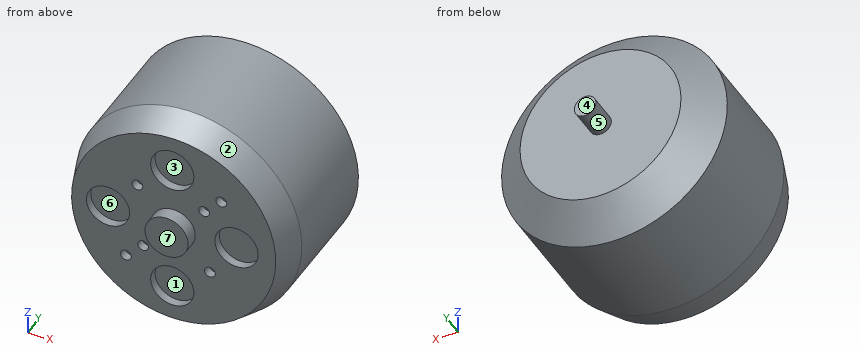
from build123d import *

# Parameters (mm, degrees)
SKETCH1_R           = 20.9
BOSS_EXTRUDE1_DEPTH = 30.75
CHAMFER1_SIZE       = 5
CHAMFER1_SIZE2      = 6
CHAMFER2_SIZE       = 2
CHAMFER2_SIZE2      = 5.494954839
SKETCH2_R           = 2
BOSS_EXTRUDE2_DEPTH = 5.5
SKETCH3_R           = 4
BOSS_EXTRUDE3_DEPTH = 2.55
SKETCH4_R           = 4
SKETCH4_R_2         = 1
CUT_EXTRUDE1_DEPTH  = 1.5875


with BuildPart() as part:
    # Sketch1 → Boss-Extrude1 (new body)
    with BuildSketch(Plane(origin=(0, 0, 0), x_dir=(1, 0, 0), z_dir=(0, 1, 0))):
        with Locations(Location((-5.649057894, -5.328088696, 0), (0, 0, 270))):
            Circle(SKETCH1_R)
    extrude(amount=BOSS_EXTRUDE1_DEPTH)

    # Chamfer1
    chamfer1_edges = [part.edges().sort_by_distance(p)[0] for p in [
        (-5.649057894, 30.75, -15.571911304),
    ]]
    chamfer1_side = [part.faces().sort_by_distance(p)[0] for p in [
        (-5.649057894, 15.375, -15.571911304),
    ]]
    chamfer(chamfer1_edges, length=CHAMFER1_SIZE, length2=CHAMFER1_SIZE2, reference=chamfer1_side[0])

    # Chamfer2
    chamfer2_edges = [part.edges().sort_by_distance(p)[0] for p in [
        (-5.649057894, 0, -15.571911304),
    ]]
    chamfer2_side = [part.faces().sort_by_distance(p)[0] for p in [
        (-5.649057894, 0, 5.328088696),
    ]]
    chamfer(chamfer2_edges, length=CHAMFER2_SIZE, length2=CHAMFER2_SIZE2, reference=chamfer2_side[0])

    # Sketch2 → Boss-Extrude2 (add)
    with BuildSketch(Plane(origin=(0, 30.75, 0), x_dir=(1, 0, 0), z_dir=(0, 1, 0))):
        with Locations(Location((-5.649057894, -5.328088696, 0), (0, 0, 270))):
            Circle(SKETCH2_R)
    extrude(amount=BOSS_EXTRUDE2_DEPTH)

    # Sketch3 → Boss-Extrude3 (add)
    with BuildSketch(Plane.XZ):
        with Locations(Location((-5.649057894, 5.328088696, 0), (0, 0, 90))):
            Circle(SKETCH3_R)
    extrude(amount=BOSS_EXTRUDE3_DEPTH)

    # Sketch4 → Cut-Extrude1 (cut)
    with BuildSketch(Plane.XZ):
        with Locations(Location((-5.908658192, 17.486035989, 0), (0, 0, 270))):
            Circle(SKETCH4_R)
        with Locations(Location((-5.908658192, -6.829858597, 0), (0, 0, 90))):
            Circle(SKETCH4_R)
        with Locations(Location((-17.807005187, 5.587688994, 0), (0, 0, 90))):
            Circle(SKETCH4_R)
        with Locations(Location((5.989688802, 5.587688994, 0), (0, 0, 270))):
            Circle(SKETCH4_R)
        with Locations(Location((-12.366572316, 12.045603117, 0), (0, 0, 270))):
            Circle(SKETCH4_R_2)
        with Locations(Location((1.068456527, -1.389425725, 0), (0, 0, 90))):
            Circle(SKETCH4_R_2)
        with Locations(Location((-11.305912144, -0.328765554, 0), (0, 0, 270))):
            Circle(SKETCH4_R_2)
        with Locations(Location((0.007796355, 10.984942945, 0), (0, 0, 90))):
            Circle(SKETCH4_R_2)
        with Locations(Location((-14.487892659, -3.510746069, 0), (0, 0, 270))):
            Circle(SKETCH4_R_2)
        with Locations(Location((3.18977687, 14.166923461, 0), (0, 0, 90))):
            Circle(SKETCH4_R_2)
    extrude(amount=-CUT_EXTRUDE1_DEPTH, mode=Mode.SUBTRACT)


solid = part.part
Verification items for the finished model (mm, model axes). Face numbers are marked on the shaded views. A direction names the side the tool comes from. Give positions to 0.01 mm unless a question says otherwise; leave off trailing zeros. Loops run counter-clockwise (first coordinate to the right, second up) from the corner with the lowest first, then second, coordinate; pieces in that order, holes last. Notation, with made-up numbers: (-17.5, 40) - (13.5, 40) arc R25 ccw to (13.5, 79) - close; hole circle Ø8 at (8.25, -17). An arc over 180 degrees is marked (long way). Write item = value, one per line. Start each with the question number.
Q1. Cross-section at B-B, the plane y = 3. Enter the section's corners in (x, z).
Q2. Tool access check on the marked faces 5, 6 and 7. Record the directions out of +Z, -Z, +X, -X, +Y, -Y that give a thin tool (end or side, any length) a straight path to the whole face; none if there is none.
Q3. Thickness scan on line 1 (Y direction, x = 2, z = 9); line 2 (Z direction, x = 6, y = 1); line 3 (X direction, y = 7.5, z = 8). Record the ranges inside material, lowest first.
Q4. Mould release check, pull along X, two halves, no side actions. Record for the marked faces 1, 2, 3 and 4: released by +X, released by -X, zero draft, split by the parting line, or undercut.
Q5. Depth check by flat-ended pin: P1, Ø1.5, axis at x = 3.5, z = -0.5, coming from the +Y side; P2, Ø1, axis at y = 8.5, z = 7, coming from the +X side; P3, Ø1.2, axis at x = 3.19, z = 14.17, coming from the -Y side. Enter the tip coordinate at first touch or a pass-through.
Q6. Cross-section at A-A, the plane y = 14.5. Enter the section's corners in (x, z), and give its area (3 significant figures).
Answer key:
q1.outline = circle Ø39.98 at (-5.65, 5.33)
q2.face_5 = +Y
q2.face_6 = -Y
q2.face_7 = +Z, -Z, +X, -X, -Y
q3.line_1 = 0 to 30.75
q3.line_2 = -10.01 to 1.59, 9.59 to 20.67
q3.line_3 = -26.38 to 15.08
q4.face_1 = undercut
q4.face_2 = split by the parting line
q4.face_3 = undercut
q4.face_4 = zero draft
q5.P1 = 30.75
q5.P2 = 15.22
q5.P3 = 1.59
q6.outline = circle Ø41.8 at (-5.65, 5.33)
q6.area = 1,370 mm^2
